For this review, take the finished solid that the model builds, in its own axes (mm). A direction names the side the tool comes from. Round coordinates to 2 decimals unless told otherwise and drop trailing zeros. Write each loop counter-clockwise with the first axis right and the second up, starting at its lowest first coordinate (ties: lowest second). Pieces come first, ordered by that corner, then holes. Notation, with made-up numbers: (46.25, -0.75) - (57.25, -0.75) arc R15 ccw to (57.25, 8.25) - close; hole circle Ø4 at (-10, 70). An arc over 180 degrees is marked (long way). One line per item, written item: value. Start each with the question number.
Q1. Add section B-B on y = 49. Write out the cut boundary in (x, z) (1 decimal).
Q2. Add section A-A on x = 14.5. Write out the cut boundary in (y, z).
Q3. Add section C-C on y = 6.5. Write out the cut boundary in (x, z) (1 decimal), and give its area (3 significant figures).
Q4. Clearance check with flat-ended pins moving along their axes: pin 1 Ø3 at (x, z) = (7.94, 12.57) entering from +Y; pin 2 Ø2 at (y, z) = (9.72, 12.57) entering from +X. State where each tip first meets the part, or that it passes through.
Q5. Mouldability with a two-part tool opening along X and no side actions: class faces 4 (the face through (9.525, 26, 10)), 5 (the face through (8.257, 13.995, 12.559)), 6 (the face through (8.05, 56.37, 24.35)) as +X half, -X half, draft (parallel to the pull), parting line (faces both ways), or undercut.
Q6. For probe 1 along Y at (x, z) = (10, 13.5); probe 2 along X at (y, z) = (13.5, 13.25) (3 decimals); probe 3 along Z at (x, y) = (5.75, 47), list the stretches that pass through material, from the lowest coordinate up.
Q7. Add section D-D on x = 3.25. Write out the cut boundary in (y, z).
Q8. Tool access review of faces 1 (the face through (12.733, 47.896, 10.733)), 2 (the face through (7.09, 45.74, 14.21)), 3 (the face through (12.6, 25.4, 17)): name each direction out of +Z, -Z, +X, -X, +Y, -Y from which nothing blocks a thin tool from reaching the whole face with its end or side.
```python
from build123d import *

# Parameters (mm, degrees)
SKETCH1_W                               = 25.146
SKETCH1_H                               = 56.769
BOSS_EXTRUDE1_DEPTH                     = 15.875
HOLE1_D                                 = 3.683
HOLE1_DEPTH                             = 12.7
HOLE1_TIP                               = 1.10648483
HOLE2_D                                 = 3.683
HOLE2_DEPTH                             = 12.7
HOLE2_TIP                               = 1.10648483
HOLE3_D                                 = 3.683
HOLE3_DEPTH                             = 23.8125
CBORE_FOR_M6_HEX_HEAD_BOLT1_D           = 6.7564
CBORE_FOR_M6_HEX_HEAD_BOLT1_CBORE_D     = 11.1252
CBORE_FOR_M6_HEX_HEAD_BOLT1_CBORE_DEPTH = 6.35
CHAMFER1_SIZE                           = 1.5748
CHAMFER2_SIZE                           = 0.254


with BuildPart() as part:
    # Sketch1 → Boss-Extrude1 (new body)
    with BuildSketch(Plane(origin=(15.875, 0, 0), x_dir=(0, 0, -1), z_dir=(1, 0, 0))):
        with Locations((-12.573, 28.7655)):
            Rectangle(SKETCH1_W, SKETCH1_H)
    extrude(amount=-BOSS_EXTRUDE1_DEPTH)

    # Hole1
    with Locations(Plane(origin=(0, 0.381, 0), x_dir=(-1, 0, 0), z_dir=(0, -1, 0))):
        with Locations((-7.9375, -12.573)):
            Hole(HOLE1_D / 2, depth=HOLE1_DEPTH)
            with Locations((0, 0, -(HOLE1_DEPTH + HOLE1_TIP / 2))):  # 118° drill point
                Cone(0, HOLE1_D / 2, HOLE1_TIP, mode=Mode.SUBTRACT)

    # Hole2
    with Locations(Plane(origin=(0, 57.15, 0), x_dir=(1, 0, 0), z_dir=(0, 1, 0))):
        with Locations((7.9375, -12.573)):
            Hole(HOLE2_D / 2, depth=HOLE2_DEPTH)
            with Locations((0, 0, -(HOLE2_DEPTH + HOLE2_TIP / 2))):  # 118° drill point
                Cone(0, HOLE2_D / 2, HOLE2_TIP, mode=Mode.SUBTRACT)

    # Hole3
    with Locations(Plane(origin=(15.875, 0, 0), x_dir=(0, 0, -1), z_dir=(1, 0, 0))):
        with Locations((-12.573, 47.8155), (-12.573, 9.7155)):
            Hole(HOLE3_D / 2, depth=HOLE3_DEPTH)

    # CBORE for M6 Hex Head Bolt1 (through all)
    with Locations(Plane(origin=(15.875, 0, 0), x_dir=(0, 0, -1), z_dir=(1, 0, 0))):
        with Locations((-12.573, 28.7655)):
            CounterBoreHole(CBORE_FOR_M6_HEX_HEAD_BOLT1_D / 2, CBORE_FOR_M6_HEX_HEAD_BOLT1_CBORE_D / 2, CBORE_FOR_M6_HEX_HEAD_BOLT1_CBORE_DEPTH)

    # Chamfer1
    chamfer1_edges = [part.edges().sort_by_distance(p)[0] for p in [
        (7.9375, 57.15, 0),
        (7.9375, 0.381, 0),
        (7.9375, 0.381, 25.146),
        (7.9375, 57.15, 25.146),
    ]]
    chamfer(chamfer1_edges, length=CHAMFER1_SIZE)

    # Chamfer2
    chamfer2_edges = [part.edges().sort_by_distance(p)[0] for p in [
        (15.875, 28.7655, 18.1356),
        (0, 28.7655, 9.1948),
    ]]
    chamfer(chamfer2_edges, length=CHAMFER2_SIZE)


solid = part.part
```
Result set:
1. outline: (0, 0) - (15.9, 0) - (15.9, 11.2) - (9.1, 11.2) arc R1.8 cw to (6.8, 11.2) - (0, 11.2) - close; (0, 14) - (6.8, 14) arc R1.8 cw to (9.1, 14) - (15.9, 14) - (15.9, 25.1) - (0, 25.1) - close
2. outline: (0.38, 1.57) - (1.96, 0) - (55.58, 0) - (57.15, 1.57) - (57.15, 23.57) - (55.58, 25.15) - (1.96, 25.15) - (0.38, 23.57) - close; hole circle Ø3.68 at (9.72, 12.57); hole circle Ø11.13 at (28.77, 12.57); hole circle Ø3.68 at (47.82, 12.57)
3. outline: (0, 0) - (15.9, 0) - (15.9, 25.1) - (0, 25.1) - close; hole circle Ø3.7 at (7.9, 12.6)
3. area: 389 mm^2
4. pin 1: stops at y = 44.25
4. pin 2: passes through
5. face 4: +X half
5. face 5: undercut
5. face 6: draft
6. probe 1: y = 0.38 to 8.12, 11.31 to 23.28, 34.25 to 46.22, 49.41 to 57.15
6. probe 2: x = 0 to 7.015, 8.86 to 15.875
6. probe 3: z = 0 to 10.92, 14.22 to 25.15
7. outline: (0.38, 1.57) - (1.96, 0) - (55.58, 0) - (57.15, 1.57) - (57.15, 23.57) - (55.58, 25.15) - (1.96, 25.15) - (0.38, 23.57) - close; hole circle Ø3.68 at (9.72, 12.57); hole circle Ø6.76 at (28.77, 12.57); hole circle Ø3.68 at (47.82, 12.57)
8. face 1: +X, -X
8. face 2: +Y
8. face 3: +X
